Study the drawing (mm; zero at the part's minimum x, y, z) and answer. A direction names the side the tool comes from. Coordinates: 2 decimals unless noted, no trailing zeros. Loops run counter-clockwise (first coordinate to the right, second up) from the corner with the lowest first, then second, coordinate; pieces in that order, holes last. Notation, with made-up numbers: (83.25, 5.5) - (142.25, 5.5) arc R31 cw to (142.25, 38.5) - close; hole circle Ø2 at (25.5, 74). An arc over 180 degrees is marked (long way). Use one line per item in the form item = value.
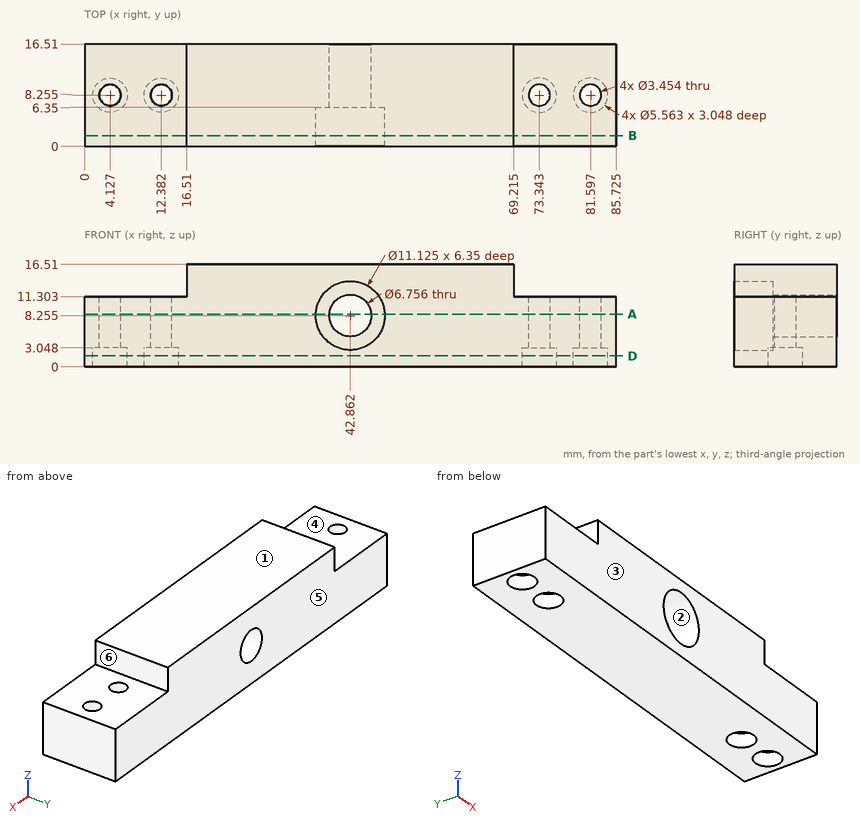
Item 1: The part is cut by section B-B on y = 1.75. Give the vertices of the cut face in (x, z) (1 decimal), plus the area to 3 significant figures.
Results below:
outline = (0, 0) - (85.7, 0) - (85.7, 11.3) - (69.2, 11.3) - (69.2, 16.5) - (16.5, 16.5) - (16.5, 11.3) - (0, 11.3) - close; hole circle Ø11.1 at (42.9, 8.3)
area = 1,150 mm²
Item 2: Find the intervals of material crossed by L1, parallel to Z at x = 40.5, y = 8.5; L2, parallel to X at y = 10.25, z = 1.5 (1 decimal); L3, parallel to X at y = 10.5, z = 8 (1 decimal), in increasing order.
Results below:
L1 = 0 to 5.84, 10.67 to 16.51
L2 = 0 to 2.2, 6.1 to 10.4, 14.3 to 71.4, 75.3 to 79.7, 83.5 to 85.7
L3 = 0 to 39.5, 46.2 to 85.7
Item 3: The part is cut by section D-D on z = 1.75. Give the vertices of the cut face in (x, y) (1 decimal).
Results below:
outline = (0, 0) - (85.7, 0) - (85.7, 16.5) - (0, 16.5) - close; hole circle Ø5.6 at (4.1, 8.3); hole circle Ø5.6 at (12.4, 8.3); hole circle Ø5.6 at (73.3, 8.3); hole circle Ø5.6 at (81.6, 8.3)
Item 4: The part is cut by section A-A on z = 8.5. Count the separate pieces of the cut face and the enclosed holes in it, plus the area to 3 significant figures.
Results below:
separate_pieces = 2
enclosed_holes = 4
area = 1,240 mm²
Item 5: Which of the six approach directions +Z, -Z, +X, -X, +Y, -Y give full straight-line access (tool end or side, diameter ignored) to the marked faces 4, 5 and 6?
Results below:
face_4 = +Z, -X, +Y, -Y
face_5 = +Z, -Z, +X, -X, +Y
face_6 = +Z, +X, +Y, -Y
Item 6: Each of these flat-tipped pins is pushed along its axis until it touches: P1, Ø1.7, axis at x = 13.5, y = 7, coming from the -Z side; P2, Ø3.5, axis at x = 43, z = 10.5, coming from the -Y side; P3, Ø5.5, axis at x = 81.6, y = 8.26, coming from the +Z side. Where does it stop, or does it pass through?
Results below:
P1 = 3.05
P2 = 6.35
P3 = 11.3
Item 7: For a pull along Z with two mould halves and no side action, classify the marked faces 1, 2 and 3 as +Z half, -Z half, draft (parallel to the pull), parting line (faces both ways), or undercut.
Results below:
face_1 = +Z half
face_2 = undercut
face_3 = draft
